from build123d import *

# Parameters (mm, degrees)
SKETCH_1_R               = 2.5
EXTRUDE_1_DEPTH          = 0.9
SKETCH_2_R               = 2.2
EXTRUDE_2_DEPTH          = 2.9
CUT_EXTRUDE_1_DEPTH      = 6.190375709
CUT_EXTRUDE_1_DEPTH_BACK = 6.190375709
SKETCH_3_R               = 1.5
SKETCH_4_W               = 0.5
SKETCH_4_H               = 8
CUT_EXTRUDE_2_DEPTH      = 2.9
SKETCH_5_W               = 2
SKETCH_5_H               = 6
CUT_EXTRUDE_3_DEPTH      = 1
SKETCH_6_R               = 2
CUT_EXTRUDE_4_DEPTH      = 1
CUT_EXTRUDE_5_DEPTH      = 6.590393546
FILLET_1_R               = 0.3
FILLET_2_R               = 0.2


with BuildPart() as part:
    # Эскиз1 → Бобышка-Вытянуть1 (new body)
    with BuildSketch(Plane.XY):
        Circle(SKETCH_1_R)
    extrude(amount=EXTRUDE_1_DEPTH)

    # Эскиз2 → Бобышка-Вытянуть2 (add)
    with BuildSketch(Plane.XY.offset(0.9)):
        Circle(SKETCH_2_R)
    extrude(amount=EXTRUDE_2_DEPTH)

    # Эскиз3 → Вырез-Вытянуть1 (cut, two sides: drawn at the far end of the back side and taken through both)
    with BuildSketch(Plane.XY.offset(3.8).offset(-CUT_EXTRUDE_1_DEPTH_BACK)):
        Circle(SKETCH_3_R)
    extrude(amount=CUT_EXTRUDE_1_DEPTH + CUT_EXTRUDE_1_DEPTH_BACK, mode=Mode.SUBTRACT)

    # Эскиз4 → Вырез-Вытянуть2 (cut)
    with BuildSketch(Plane.XY.offset(3.8)):
        with Locations((-1, 0)):
            Rectangle(SKETCH_4_W, SKETCH_4_H)
        with Locations((1, 0)):
            Rectangle(SKETCH_4_W, SKETCH_4_H)
    extrude(amount=-CUT_EXTRUDE_2_DEPTH, mode=Mode.SUBTRACT)

    # Эскиз5 → Вырез-Вытянуть3 (cut)
    with BuildSketch(Plane.XY.offset(3.8)):
        with Locations((-2.25, -1.189613301)):
            Rectangle(SKETCH_5_W, SKETCH_5_H)
        with Locations((2.25, -1.189613301)):
            Rectangle(SKETCH_5_W, SKETCH_5_H)
    extrude(amount=-CUT_EXTRUDE_3_DEPTH, mode=Mode.SUBTRACT)

    # Эскиз6 → Вырез-Вытянуть4 (cut)
    with BuildSketch(Plane.XY.offset(2.8)):
        Circle(SKETCH_6_R)
    extrude(amount=-CUT_EXTRUDE_4_DEPTH, mode=Mode.SUBTRACT)

    # Эскиз7 → Вырез-Вытянуть5 (cut, through all)
    with BuildSketch(Plane.ZY.offset(0.75)):
        Polygon((3.8, 1.683624947), (2.8, 1.299038106), (3.8, 1.299038106), align=None)
        Polygon((3.8, -1.683624947), (2.8, -1.299038106), (3.8, -1.299038106), align=None)
    extrude(amount=-CUT_EXTRUDE_5_DEPTH, mode=Mode.SUBTRACT)

    # Скругление1
    fillet_1_edges = [part.edges().sort_by_distance(p)[0] for p in [
        (-1.5, 0, 0),
        (-2.5, 0, 0),
    ]]
    fillet(fillet_1_edges, radius=FILLET_1_R)

    # Скругление2
    fillet_2_edges = [part.edges().sort_by_distance(p)[0] for p in [
        (1.436140662, 0.433012702, 1.8),
        (0, -1.5, 1.8),
        (0, 1.5, 1.8),
        (-1.5, 0, 1.8),
        (0, 2.2, 3.8),
        (0, -2.2, 3.8),
        (2.2, 0, 2.8),
        (-2.2, 0, 2.8),
    ]]
    fillet(fillet_2_edges, radius=FILLET_2_R - 0.0001)  # a hair under: the kernel refuses the full size


solid = part.part
For this review, take the finished solid that the model builds, in its own axes (mm). A direction names the side the tool comes from. Round coordinates to 2 decimals unless told otherwise and drop trailing zeros. Order: outer loops, then holes, each group sorted by start corner. A loop starts at its lowest first (then second) coordinate and runs counter-clockwise, first axis right, second up. Notation, with made-up numbers: M -8.5,76 L 43.5,76 A26 cw 43.5,112 Z; hole C -9,-8.5 d7. An arc over 180 degrees is marked long. Write each question's results on one line, items separated by ' | '. Start each with the question number.
1. Draft analysis for pull direction X (two halves, no side actions). For faces 5 (the face through (1.386, -0.575, 0.941)), 6 (the face through (-2.2, 0, 1.7)), 7 (the face through (2.2, 0, 1.7)), 8 (the face through (0, -2.2, 2.2)), state which applies: pulls with the +X half, pulls with the -X half, needs draft (parallel to the pull), parting line crosses it, or undercut.
2. Add section C-C (y = 1.4). State how many separate pieces and enclosed holes the cut face has, then the cut area to 3 significant figures.
3. Tool access review of faces 1 (the face through (0, 2, 2)), 2 (the face through (-0.9, -1.5, 0.9)), 3 (the face through (-0.01, 1.58, 3.53)), 4 (the face through (1.25, 1.4, 1.4)): name each direction out of +Z, -Z, +X, -X, +Y, -Y from which nothing blocks a thin tool from reaching the whole face with its end or side.
4. Add section B-B (z = 0.75). State the section outline as (x, y) points, then the cut area to 3 significant figures.
5. To check wall thickness, follow L1, parallel to X at y = -1.55, z = 1.3; L2, parallel to X at y = 0, z = 1.1; L3, parallel to Y at x = 0, z = 0.75. State the ranges of each line that lie inside material, in increasing order. Write a range as [from, to].
6. Clearance check with flat-ended pins moving along their axes: pin 1 Ø0.8 at (y, z) = (2, 1.5) entering from +X; pin 2 Ø0.8 at (x, y) = (0, 1.5) entering from -Z; pin 3 Ø0.5 at (y, z) = (-1.5, 2) entering from +X; pin 4 Ø0.5 at (y, z) = (1.5, 2) entering from -X. State where each tip first meets the part, or that it passes through.
Output values:
1) face 5: undercut | face 6: pulls with the -X half | face 7: pulls with the +X half | face 8: parting line crosses it
2) separate pieces: 4 | enclosed holes: 0 | area: 4.40 mm^2
3) face 1: none | face 2: +Z | face 3: +Z, +X, -X | face 4: +Z, +Y, -Y
4) outline: C 0,0 d5; hole C 0,0 d3 | area: 12.6 mm^2
5) L1: [-1.56, -1.25], [-0.75, 0.75], [1.25, 1.56] | L2: [-2.2, -1.5], [1.5, 2.2] | L3: [-2.5, -1.5], [1.5, 2.5]
6) pin 1: x = 1.51 | pin 2: z = 0 | pin 3: x = 1.81 | pin 4: x = -1.81
